Job drawing, mm, ordinate dimensions from the low corner. One solid piece. A direction names the side the tool comes from. Give positions to 0.01 mm unless a question says otherwise; leave off trailing zeros. Order: outer loops, then holes, each group sorted by start corner. A loop starts at its lowest first (then second) coordinate and runs counter-clockwise, first axis right, second up. Notation, with made-up numbers: (55.5, 39) - (104.5, 39) arc R18 cw to (104.5, 47) - close; hole circle Ø7 at (8.25, 39.5). An arc over 180 degrees is marked (long way). One line per item, written item: value.
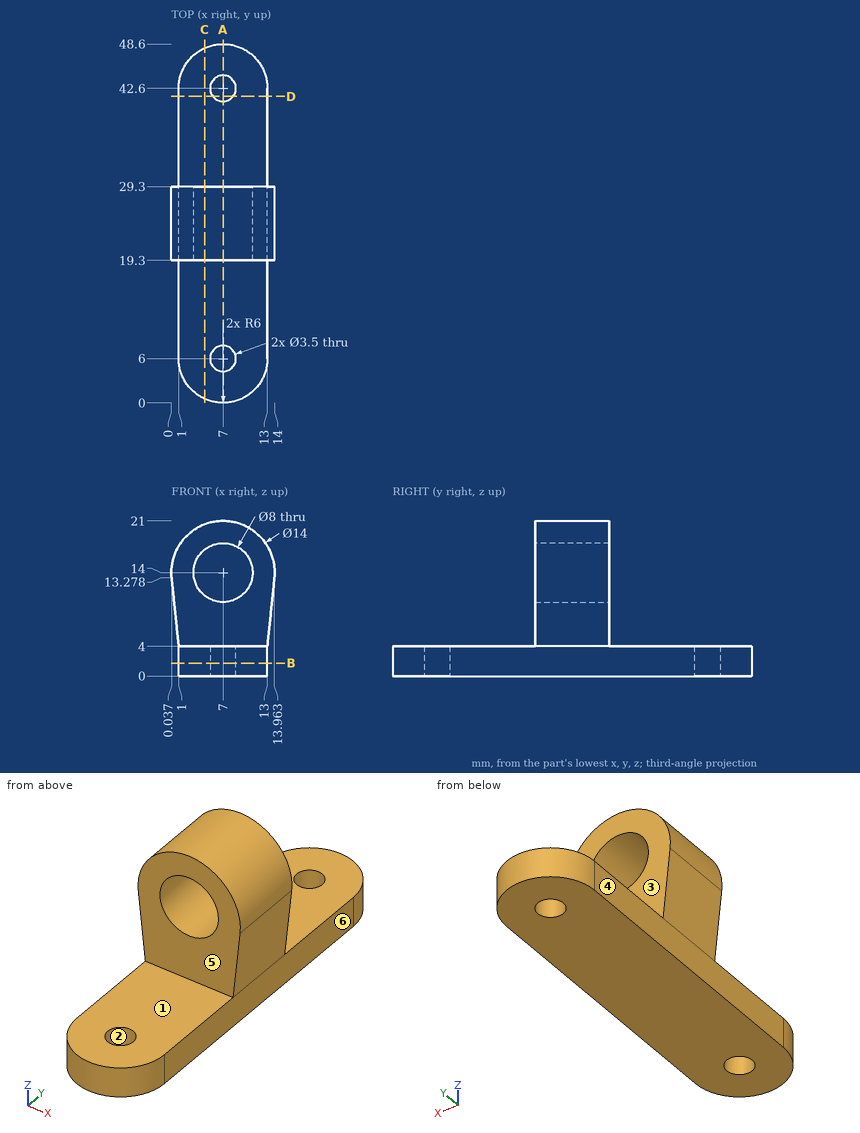
1) Slice it at D-D on y = 41.5. Write the cut outline in (x, z), then the cut area to 3 significant figures.
Answer:
outline: (1, 0) - (5.64, 0) - (5.64, 4) - (1, 4) - close; (8.36, 0) - (13, 0) - (13, 4) - (8.36, 4) - close
area: 37.1 mm2
2) Slice it at A-A on x = 7. Write the cut outline in (y, z).
Answer:
outline: (0, 0) - (4.25, 0) - (4.25, 4) - (0, 4) - close; (7.75, 0) - (40.85, 0) - (40.85, 4) - (29.3, 4) - (29.3, 10) - (19.3, 10) - (19.3, 4) - (7.75, 4) - close; (19.3, 18) - (29.3, 18) - (29.3, 21) - (19.3, 21) - close; (44.35, 0) - (48.6, 0) - (48.6, 4) - (44.35, 4) - close
3) Slice it at B-B on z = 1.75. Write the cut outline in (x, y), then the cut area to 3 significant figures.
Answer:
outline: (1, 6) arc R6 ccw to (13, 6) - (13, 42.6) arc R6 ccw to (1, 42.6) - close; hole circle Ø3.5 at (7, 6); hole circle Ø3.5 at (7, 42.6)
area: 533 mm2
4) Two-plate mould, pull along Y, no slides. Class the marked faces 1, 2 and 3: pulls with the +Y half, pulls with the -Y half, needs draft (parallel to the pull), parting line crosses it, or undercut.
Answer:
face 1: needs draft
face 2: undercut
face 3: pulls with the +Y half
5) Drop flat-ended pins along their axis: P1, Ø6, axis at x = 4.5, y = 8, coming from the +Z side; P2, Ø5, axis at y = 14.5, z = 10.5, coming from the +X side; P3, Ø4, axis at x = 8.5, z = 16, coming from the -Y side; P4, Ø4.5, axis at y = 24.5, z = 2.5, coming from the -X side. Give the stop position or say it passes through.
Answer:
P1: stops at z = 4
P2: passes through
P3: stops at y = 19.3
P4: stops at x = 0.92
6) Wall check: line 1 along Y through (x, z) = (7, 1); line 2 along X through (y, z) = (24.25, 14); line 3 along Y through (x, z) = (8, 2.5) (1 decimal). Give the ranges that are in metal, low to high. Write a range as [from, to].
Answer:
line 1: y = [0, 4.25], [7.75, 40.85], [44.35, 48.6]
line 2: x = [0, 3], [11, 14]
line 3: y = [0.1, 4.6], [7.4, 41.2], [44, 48.5]
7) Which spindle directions (+Z, -Z, +X, -X, +Y, -Y) get a long thin tool onto all of the face, cutting with end or side? Do the marked faces 4, 5 and 6. Say none if no direction does.
Answer:
face 4: -Z, -X, +Y, -Y
face 5: +Z, +X, -X, -Y
face 6: -Z, +X, +Y, -Y
8) Slice it at C-C on x = 4.5. Write the cut outline in (y, z) (1 decimal).
Answer:
outline: (0.5, 0) - (48.1, 0) - (48.1, 4) - (29.3, 4) - (29.3, 10.9) - (19.3, 10.9) - (19.3, 4) - (0.5, 4) - close; (19.3, 17.1) - (29.3, 17.1) - (29.3, 20.5) - (19.3, 20.5) - close
